The listing builds one solid part. Answer for the finished solid, in the listing's coordinates (mm). Face numbers are marked on the shaded views. A direction names the side the tool comes from. Coordinates: 2 decimals unless noted, no trailing zeros. Order: outer loops, then holes, each group sorted by start corner. A loop starts at its lowest first (then second) coordinate and runs counter-clockwise, first axis right, second up. Notation, with made-up numbers: (-7, -24) - (34, -24) arc R16 ccw to (34, -18) - close; hole circle Ø6 at (-35, 2.25). An arc over 180 degrees is marked (long way). Use one line per item in the form item = value. Start each with the question number.
Item 1: Each of these flat-tipped pins is pushed along its axis until it touches: pin 1 Ø2 at (x, y) = (-0.5, 13) entering from +Z; pin 2 Ø1.5 at (x, z) = (-1, 16.5) entering from +Y; pin 3 Ø5 at (y, z) = (12.5, 32) entering from +X. Where does it stop, or does it pass through?
Item 2: Section A-A, the plane z = 12 is taken. Write down the section's boundary in (x, y).
Item 3: Section B-B, the plane y = 10 is taken. Write down the section's boundary in (x, z).
Item 4: Section D-D, the plane z = 37 is taken. Write down the section's boundary in (x, y).
Item 5: A tool of negligible diameter and unlimited length cuts with its end or side. For the marked faces 1 and 2, from which of +Z, -Z, +X, -X, +Y, -Y can it reach the whole face along a straight path? Write none if from no direction.
Item 6: Section C-C, the plane x = 2.5 is taken. Write down the section's boundary in (y, z), and give its area (3 significant figures).
Item 7: Consider line 1 along X through (y, z) = (2.1, 12); line 2 along X through (y, z) = (9.5, 12); line 3 along Y through (x, z) = (4.25, 10). Determine where each line is inside the solid, lowest interval first. Write a range as [from, to].
from build123d import *

# Parameters (mm, degrees)
EXTRUDE_1_DEPTH     = 45
SKETCH_3_R          = 1.5
CUT_EXTRUDE_1_DEPTH = 50.738044303
SKETCH_2_R          = 1.5
CUT_EXTRUDE_2_DEPTH = 51.68530359
CUT_EXTRUDE_3_DEPTH = 50.738044303


with BuildPart() as part:
    # 草图1 → 凸台-拉伸1 (new body)
    with BuildSketch(Plane.XY):
        Polygon((-2.009073658, 20), (-2.009073658, 3), (6.990926342, 3), (6.990926342, 0), (-5.009073658, 0), (-5.009073658, 20), align=None)
    extrude(amount=EXTRUDE_1_DEPTH)

    # 草图3 → 切除-拉伸1 (cut, through all)
    with BuildSketch(Plane.XZ):
        with Locations((1.990926342, 33)):
            Circle(SKETCH_3_R)
        with Locations(Location((1.990926342, 12, 0), (0, 0, 270))):
            Circle(SKETCH_3_R)
    extrude(amount=-CUT_EXTRUDE_1_DEPTH, mode=Mode.SUBTRACT)

    # 草图2 → 切除-拉伸2 (cut, through all)
    with BuildSketch(Plane.ZY.offset(5.009073658)):
        with Locations((4, 10)):
            Circle(SKETCH_2_R)
        with Locations(Location((41, 10, 0), (0, 0, 270))):
            Circle(SKETCH_2_R)
    extrude(amount=-CUT_EXTRUDE_2_DEPTH, mode=Mode.SUBTRACT)

    # 草图4 → 切除-拉伸3 (cut, through all)
    with BuildSketch(Plane.XZ):
        Polygon((-0.009073658, 45), (6.990926342, 38), (6.990926342, 45), align=None)
        Polygon((6.990926342, 7), (6.990926342, 0), (-0.009073658, 0), align=None)
    extrude(amount=-CUT_EXTRUDE_3_DEPTH, mode=Mode.SUBTRACT)


solid = part.part
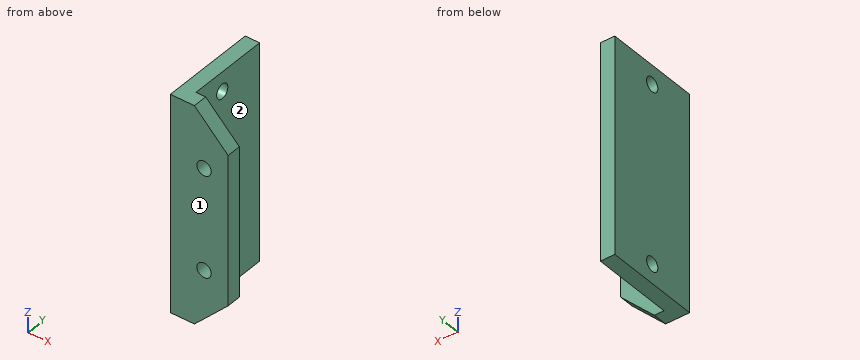
Response:
q1.pin_1 = through
q1.pin_2 = 3
q1.pin_3 = -2.01
q2.outline = (-5.01, 0) - (0.49, 0) - (0.49, 3) - (-2.01, 3) - (-2.01, 20) - (-5.01, 20) - close; (3.49, 0) - (6.99, 0) - (6.99, 3) - (3.49, 3) - close
q3.outline = (-5.01, 0) - (-2.01, 0) - (-2.01, 2.5) - (-5.01, 2.5) - close; (-5.01, 5.5) - (-2.01, 5.5) - (-2.01, 39.5) - (-5.01, 39.5) - close; (-5.01, 42.5) - (-2.01, 42.5) - (-2.01, 45) - (-5.01, 45) - close
q4.outline = (-5.01, 0) - (6.99, 0) - (6.99, 3) - (-2.01, 3) - (-2.01, 20) - (-5.01, 20) - close
q5.face_1 = +Z, -Z, +X, -X, -Y
q5.face_2 = +Z, -Z, +X, +Y
q6.outline = (0, 2.51) - (3, 2.51) - (3, 10.59) - (0, 10.59) - close; (0, 13.41) - (3, 13.41) - (3, 31.59) - (0, 31.59) - close; (0, 34.41) - (3, 34.41) - (3, 42.49) - (0, 42.49) - close
q6.area = 103 mm2
q7.line_1 = [-5.01, 0.49], [3.49, 6.99]
q7.line_2 = [-5.01, -2.01]
q7.line_3 = [0, 3]
